from build123d import *

# Parameters (mm, degrees)
F0_W     = 11
F0_H     = 65
F3_DEPTH = 19
F4_DEPTH = 65
F5_DEPTH = 65.001
F6_R     = 1.2
F7_R     = 1.99999
F2_R     = 2.5
F2_R_2   = 4
F2_R_3   = 3
F2_R_4   = 2
F8_DEPTH = 65.001


# Not quite as in the source:
# - a fillet or chamfer is up to 0.001 mm smaller than in the source, because OpenCascade refuses the exact size
# - a feature names something its author has since deleted; it is built from what else it names


with BuildPart() as f1:
    # F0 (on Front) → F1 (revolve)
    with BuildSketch(Plane.XZ):
        with Locations((-23.5, 0)):
            Rectangle(F0_W, F0_H)
    revolve(axis=Axis((0, 0, 0.8657751605), (0, 0, -1)))

    # F2 (on face) → F3 (cut)
    with BuildSketch(Plane.XY.offset(32.5)):
        with BuildLine():
            ThreePointArc((-4.5, 22.9), (0, 27.4), (4.5, 22.9))
            Line((4.5, 22.9), (4.5, 17.4284250579))
            ThreePointArc((4.5, 17.4284250579), (5.7655124222, 17.0516528967), (7, 16.5831239518))
            Line((7, 16.5831239518), (5.5, 28.4736720498))
            Line((5.5, 28.4736720498), (-5.5, 28.4736720498))
            Line((-5.5, 28.4736720498), (-7, 16.5831239518))
            ThreePointArc((-7, 16.5831239518), (-5.7655124222, 17.0516528967), (-4.5, 17.4284250579))
            Line((-4.5, 17.4284250579), (-4.5, 22.9))
        make_face()
        with BuildLine():
            Line((-5.5, 28.4736720498), (5.5, 28.4736720498))
            ThreePointArc((5.5, 28.4736720498), (0, 29), (-5.5, 28.4736720498))
        make_face()
        with BuildLine():
            ThreePointArc((17.6540730561, -3.5119374324), (12.7279220614, -12.7279220614), (3.5119374324, -17.6540730561))
            Line((3.5119374324, -17.6540730561), (8.4852813742, -22.627416998))
            Line((8.4852813742, -22.627416998), (5.6568542495, -25.4558441227))
            Line((5.6568542495, -25.4558441227), (2.1959599702, -28.916738402))
            ThreePointArc((2.1959599702, -28.916738402), (20.5060966544, -20.5060966544), (28.916738402, -2.1959599702))
            Line((28.916738402, -2.1959599702), (25.4558441227, -5.6568542495))
            Line((25.4558441227, -5.6568542495), (22.627416998, -8.4852813742))
            Line((22.627416998, -8.4852813742), (17.6540730561, -3.5119374324))
        make_face()
    extrude(amount=-F3_DEPTH, mode=Mode.SUBTRACT)

    # F2 (on face) → F4 (join, through all)
    with BuildSketch(Plane.XY.offset(32.5)):
        Polygon((8.4852813742, -22.627416998), (3.5119374324, -17.6540730561), (0.6835103076, -20.4825001809), (5.6568542495, -25.4558441227), align=None)
        with BuildLine():
            Line((5.6568542495, -25.4558441227), (0.6835103076, -20.4825001809))
            Line((0.6835103076, -20.4825001809), (-6.981162826, -28.1471733145))
            ThreePointArc((-6.981162826, -28.1471733145), (-2.4233446306, -28.8985709128), (2.1959599702, -28.916738402))
            Line((2.1959599702, -28.916738402), (5.6568542495, -25.4558441227))
        make_face()
        with BuildLine():
            ThreePointArc((2.1959599702, -28.916738402), (-2.4233446306, -28.8985709128), (-6.981162826, -28.1471733145))
            Line((-6.981162826, -28.1471733145), (-2.0078188841, -33.1205172564))
            Line((-2.0078188841, -33.1205172564), (2.1959599702, -28.916738402))
        make_face()
        Polygon((25.4558441227, -5.6568542495), (20.4825001809, -0.6835103076), (17.6540730561, -3.5119374324), (22.627416998, -8.4852813742), align=None)
        with BuildLine():
            Line((28.1471733145, 6.981162826), (20.4825001809, -0.6835103076))
            Line((20.4825001809, -0.6835103076), (25.4558441227, -5.6568542495))
            Line((25.4558441227, -5.6568542495), (28.916738402, -2.1959599702))
            ThreePointArc((28.916738402, -2.1959599702), (28.9791771248, -1.0987689344), (29, 0))
            ThreePointArc((29, 0), (28.7860037702, 3.5165305259), (28.1471733145, 6.981162826))
        make_face()
        with BuildLine():
            Line((33.1205172564, 2.0078188841), (28.1471733145, 6.981162826))
            ThreePointArc((28.1471733145, 6.981162826), (28.7860037702, 3.5165305259), (29, 0))
            ThreePointArc((29, 0), (28.9791771248, -1.0987689344), (28.916738402, -2.1959599702))
            Line((28.916738402, -2.1959599702), (33.1205172564, 2.0078188841))
        make_face()
    extrude(amount=-F4_DEPTH)

    # F2 (on face) → F5 (cut, through all)
    with BuildSketch(Plane.XY.offset(32.5)):
        with BuildLine():
            ThreePointArc((-4.5, 22.9), (0, 18.4), (4.5, 22.9))
            ThreePointArc((4.5, 22.9), (0, 27.4), (-4.5, 22.9))
        make_face()
        with BuildLine():
            Line((4.5, 17.4284250579), (4.5, 22.9))
            ThreePointArc((4.5, 22.9), (0, 18.4), (-4.5, 22.9))
            Line((-4.5, 22.9), (-4.5, 17.4284250579))
            ThreePointArc((-4.5, 17.4284250579), (0, 18), (4.5, 17.4284250579))
        make_face()
        with BuildLine():
            ThreePointArc((7, 16.5831239518), (5.7655124222, 17.0516528967), (4.5, 17.4284250579))
            ThreePointArc((4.5, 17.4284250579), (0, 18), (-4.5, 17.4284250579))
            ThreePointArc((-4.5, 17.4284250579), (-5.7655124222, 17.0516528967), (-7, 16.5831239518))
            Line((-7, 16.5831239518), (7, 16.5831239518))
        make_face()
        with BuildLine():
            ThreePointArc((28.1471733145, 6.981162826), (19.9628418868, 21.0353260921), (5.5, 28.4736720498))
            ThreePointArc((5.5, 28.4736720498), (18.4372066045, 16.6935009467), (20.4825001809, -0.6835103076))
            Line((20.4825001809, -0.6835103076), (28.1471733145, 6.981162826))
        make_face()
        with BuildLine():
            ThreePointArc((17.6540730561, -3.5119374324), (12.7279220614, -12.7279220614), (3.5119374324, -17.6540730561))
            Line((3.5119374324, -17.6540730561), (8.4852813742, -22.627416998))
            Line((8.4852813742, -22.627416998), (5.6568542495, -25.4558441227))
            Line((5.6568542495, -25.4558441227), (2.1959599702, -28.916738402))
            ThreePointArc((2.1959599702, -28.916738402), (20.5060966544, -20.5060966544), (28.916738402, -2.1959599702))
            Line((28.916738402, -2.1959599702), (25.4558441227, -5.6568542495))
            Line((25.4558441227, -5.6568542495), (22.627416998, -8.4852813742))
            Line((22.627416998, -8.4852813742), (17.6540730561, -3.5119374324))
        make_face()
        with BuildLine():
            Line((28.1471733145, 6.981162826), (20.4825001809, -0.6835103076))
            Line((20.4825001809, -0.6835103076), (25.4558441227, -5.6568542495))
            Line((25.4558441227, -5.6568542495), (28.916738402, -2.1959599702))
            ThreePointArc((28.916738402, -2.1959599702), (28.9791771248, -1.0987689344), (29, 0))
            ThreePointArc((29, 0), (28.7860037702, 3.5165305259), (28.1471733145, 6.981162826))
        make_face()
        with BuildLine():
            Line((33.1205172564, 2.0078188841), (28.1471733145, 6.981162826))
            ThreePointArc((28.1471733145, 6.981162826), (28.7860037702, 3.5165305259), (29, 0))
            ThreePointArc((29, 0), (28.9791771248, -1.0987689344), (28.916738402, -2.1959599702))
            Line((28.916738402, -2.1959599702), (33.1205172564, 2.0078188841))
        make_face()
        with BuildLine():
            Line((5.6568542495, -25.4558441227), (0.6835103076, -20.4825001809))
            Line((0.6835103076, -20.4825001809), (-6.981162826, -28.1471733145))
            ThreePointArc((-6.981162826, -28.1471733145), (-2.4233446306, -28.8985709128), (2.1959599702, -28.916738402))
            Line((2.1959599702, -28.916738402), (5.6568542495, -25.4558441227))
        make_face()
        with BuildLine():
            Line((-6.981162826, -28.1471733145), (0.6835103076, -20.4825001809))
            ThreePointArc((0.6835103076, -20.4825001809), (-16.6935009467, -18.4372066045), (-28.4736720498, -5.5))
            ThreePointArc((-28.4736720498, -5.5), (-21.0353260921, -19.9628418868), (-6.981162826, -28.1471733145))
        make_face()
        with BuildLine():
            ThreePointArc((2.1959599702, -28.916738402), (-2.4233446306, -28.8985709128), (-6.981162826, -28.1471733145))
            Line((-6.981162826, -28.1471733145), (-2.0078188841, -33.1205172564))
            Line((-2.0078188841, -33.1205172564), (2.1959599702, -28.916738402))
        make_face()
    extrude(amount=-F5_DEPTH, mode=Mode.SUBTRACT)

    # F6
    f6_edges = [f1.edges().sort_by_distance(p)[0] for p in [
        (3.511937, -17.654073, 0),
        (4.5, 17.428425, -9.5),
        (7, 16.583124, 23),
        (-7, 16.583124, 23),
        (-4.5, 17.428425, -9.5),
        (5.5, 28.473672, 23),
        (-5.5, 28.473672, 23),
        (0.68351, -20.4825, 0),
        (20.4825, -0.68351, 0),
        (17.654073, -3.511937, 0),
    ]]
    fillet(f6_edges, radius=F6_R)

    # F7 (radius 2 in the source; OpenCascade refuses exactly that, so slightly less here)
    f7_edges = [f1.edges().sort_by_distance(p)[0] for p in [
        (5.656854, -25.455844, 0),
        (8.485281, -22.627417, 0),
        (22.627417, -8.485281, 0),
        (25.455844, -5.656854, 0),
    ]]
    fillet(f7_edges, radius=F7_R)

    # F2 (on face) → F8 (cut, through all)
    with BuildSketch(Plane.XY.offset(32.5)):
        with Locations((-9.916601295, 20.7523738102)):
            Circle(F2_R)
        with Locations((-16.2634559673, 16.2634559673)):
            Circle(F2_R_2)
        with Locations((-21.397117557, 8.4358378511)):
            Circle(F2_R_2)
        with Locations((10.6623319362, 20.3792707839)):
            Circle(F2_R_3)
        with Locations((-22.9898786685, -0.6822600723)):
            Circle(F2_R_2)
        with Locations((-21.2449889591, -8.8119489404)):
            Circle(F2_R_3)
        with Locations((-16.2738828113, -14.2753784675)):
            Circle(F2_R_4)
        with Locations((15.4069372375, 14.9056833158)):
            Circle(F2_R_4)
    extrude(amount=-F8_DEPTH, mode=Mode.SUBTRACT)


solid = f1.part
Input: part model. Units: mm. Frame: model coordinates. A direction names the side the tool comes from. Round coordinates to 2 decimals unless told otherwise and drop trailing zeros. Order: outer loops, then holes, each group sorted by start corner. A loop starts at its lowest first (then second) coordinate and runs counter-clockwise, first axis right, second up. Notation, with made-up numbers: (57, 84) - (107, 84) arc R31 cw to (107, 119) - close; hole circle Ø9 at (72, 66.25). An arc over 180 degrees is marked (long way). Answer as a JSON object with one key per item and string values. Group by question number.
(1) Pin query (flat end, axial travel): P1, Ø7, axis at x = -22.99, y = -0.68, coming from the +Z side; P2, Ø1.5, axis at x = -4, z = 1, coming from the +Y side; P3, Ø9, axis at x = -21.4, y = 8.44, coming from the +Z side; P4, Ø5, axis at y = -14, z = 7.5, coming from the -X side. Return the tip coordinate at first contact, or that it passes through.
(2) Cut plane A-A (z = 23.5). Count the separate pieces of the cut face and the enclosed holes in it, then the cut area to 3 significant figures.
(3) Reachability of faces 1 (the face through (-4.5, 21, -9)), 2 (the face through (-1.2, 27.4, 13.5)), 3 (the face through (19.68, -5.54, 0.45)), 4 (the face through (5.49, -19.63, 0.45)) from +Z, -Z, +X, -X, +Y, -Y: full face, straight path, thin tool, end or side. Return the list, or none.
(4) Draft query along X for faces 5 (the face through (7.657, -22.649, 0.455)), 6 (the face through (6.35, 21.74, 23.13)), 7 (the face through (5.635, -24.627, 0.455)). Return one class per face: released by +X, released by -X, zero draft, split by the parting line, or undercut.
(5) Material intervals for probe 1 along Y at (x, z) = (-12, 25); probe 2 along X at (y, z) = (-4, -18); probe 3 along X at (y, z) = (6.5, 26.5), sorted ascending. Write a range as from..to.
(6) Cut plane B-B (x = 10). Return loops of the section in (y, z).
Here are the results:
{
 "1": {"P1": "passes through", "P2": "stops at y = 28.82", "P3": "stops at z = 32.5", "P4": "stops at x = -25.04"},
 "2": {"separate pieces": "2", "enclosed holes": "8", "area": "575 mm^2"},
 "3": {"face 1": "+Z, -Z", "face 2": "+Z", "face 3": "+Z, -Z, -Y", "face 4": "+Z, -Z, +X"},
 "4": {"face 5": "released by +X", "face 6": "undercut", "face 7": "split by the parting line"},
 "5": {"probe 1": "y = -20.28..-13.42, 13.42..19.37, 22.13..26.4", "probe 2": "x = -28.72..-25.22, -20.76..-17.55, 18.14..23.8", "probe 3": "x = -28.26..-24.9, -17.9..-16.79, 16.79..21.17"},
 "6": {"outline": "(14.97, -32.5) - (17.45, -32.5) - (17.45, 32.5) - (14.97, 32.5) - close; (23.31, -32.5) - (26.11, -32.5) - (26.11, 32.5) - (23.31, 32.5) - close"}
}
